```python
from build123d import *

# Parameters (mm, degrees)
SKETCH2_W                = 20
SKETCH2_H                = 5
BOSS_EXTRUDE1_DEPTH      = 10
SKETCH4_R                = 2
BOSS_EXTRUDE2_DEPTH      = 3.333333333
BOSS_EXTRUDE3_START      = -3.333333333
SKETCH5_R                = 2
BOSS_EXTRUDE3_DEPTH      = 3.333333333
BOSS_EXTRUDE4_DEPTH      = 1.5
BOSS_EXTRUDE4_DEPTH_BACK = 1.5
SKETCH7_R                = 2
BOSS_EXTRUDE5_DEPTH      = 1.5
BOSS_EXTRUDE5_DEPTH_BACK = 1.5
CUT_EXTRUDE1_DEPTH       = 27.57654043


with BuildPart() as part:
    # Sketch2 → Boss-Extrude1 (new body)
    with BuildSketch(Plane(origin=(0, 0, 0), x_dir=(0, 0, -1), z_dir=(1, 0, 0))):
        with Locations((10, 2.5)):
            Rectangle(SKETCH2_W, SKETCH2_H)
    extrude(amount=BOSS_EXTRUDE1_DEPTH)

    # Sketch4 → Boss-Extrude2 (add)
    with BuildSketch(Plane(origin=(10, 0, 0), x_dir=(0, 0, -1), z_dir=(1, 0, 0))):
        with BuildLine():
            Line((-2.5, 5), (0, 5))
            Line((0, 5), (0, 2.5))
            ThreePointArc((0, 2.5), (-4.267766953, 0.732233047), (-2.5, 5))
        make_face()
        with Locations((-2.5, 2.5)):
            Circle(SKETCH4_R, mode=Mode.SUBTRACT)
    extrude(amount=-BOSS_EXTRUDE2_DEPTH)

    # Sketch5 → Boss-Extrude3 (add)
    with BuildSketch(Plane.ZY.offset(BOSS_EXTRUDE3_START)):
        with BuildLine():
            Line((2.5, 5), (0, 5))
            Line((0, 5), (0, 2.5))
            ThreePointArc((0, 2.5), (4.267766953, 0.732233047), (2.5, 5))
        make_face()
        with Locations(Location((2.5, 2.5, 0), (0, 0, 180))):
            Circle(SKETCH5_R, mode=Mode.SUBTRACT)
    extrude(amount=BOSS_EXTRUDE3_DEPTH)

    # Sketch7 → Boss-Extrude4 (add, two sides: drawn at the far end of the back side and taken through both)
    with BuildSketch(Plane(origin=(5, 0, 0), x_dir=(0, 0, -1), z_dir=(1, 0, 0)).offset(-BOSS_EXTRUDE4_DEPTH_BACK)):
        with BuildLine():
            Line((20, 5), (22.5, 5))
            ThreePointArc((22.5, 5), (24.267766953, 0.732233047), (20, 2.5))
            Line((20, 2.5), (20, 5))
        make_face()
        with Locations((22.5, 2.5)):
            Circle(SKETCH7_R, mode=Mode.SUBTRACT)
    extrude(amount=BOSS_EXTRUDE4_DEPTH + BOSS_EXTRUDE4_DEPTH_BACK)

    # Sketch8 → Boss-Extrude5 (add, two sides: drawn at the far end of the back side and taken through both)
    with BuildSketch(Plane(origin=(5, 0, 0), x_dir=(0, 0, -1), z_dir=(1, 0, 0)).offset(-BOSS_EXTRUDE5_DEPTH_BACK)):
        with BuildLine():
            Line((0, 5), (2, 5))
            Line((2, 5), (5.2, 5))
            Line((5.2, 5), (5.2, 5.04))
            add(Edge.make_bspline(
                [(2, 6.25), (2.633677282, 6.25), (3.485069852, 5.13334343), (4.685132782, 5.04), (5.2, 5.04)],
                knots=[0, 0, 0, 0, 0.555540961, 1, 1, 1, 1], degree=3))
            Line((2, 6.25), (-8, 6.25))
            Line((-8, 6.25), (-8, 5))
            Line((-8, 5), (0, 5))
        make_face()
    extrude(amount=BOSS_EXTRUDE5_DEPTH + BOSS_EXTRUDE5_DEPTH_BACK)

    # Sketch9 → Cut-Extrude1 (cut, through all)
    with BuildSketch(Plane.ZY.offset(-3.5)):
        Polygon((8, 6.25), (5.838024107, 6.25), (5.838024107, 5.183121739), (2.5, 5.183121739), (2.5, 5), (8, 5), align=None)
    extrude(amount=-CUT_EXTRUDE1_DEPTH, mode=Mode.SUBTRACT)


solid = part.part
```
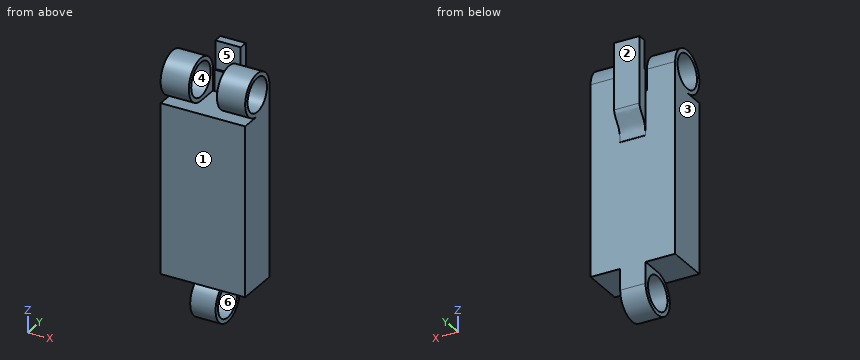
The model under review builds one solid part; all positions refer to its coordinate system, in mm. Face numbers are marked on the shaded views. A direction names the side the tool comes from. Give positions to 0.01 mm unless a question says otherwise; leave off trailing zeros. Write each loop counter-clockwise with the first axis right and the second up, starting at its lowest first coordinate (ties: lowest second). Pieces come first, ordered by that corner, then holes. Notation, with made-up numbers: (57.5, 72.5) -> (76.5, 72.5) arc R14 ccw to (76.5, 80.5) -> close; hole circle Ø6 at (85, -14). An arc over 180 degrees is marked (long way). Answer in a Markdown table with one row per item.
1) Add section A-A on y = 4. State the section outline as (x, z) points.
Worked answers:
| item | result |
|---|---|
| outline | (0, -20) -> (3.5, -20) -> (3.5, -21.18) -> (6.5, -21.18) -> (6.5, -20) -> (10, -20) -> (10, 1.18) -> (6.67, 1.18) -> (6.67, 0) -> (3.33, 0) -> (3.33, 1.18) -> (0, 1.18) -> close; (0, 3.82) -> (3.33, 3.82) -> (3.33, 4.5) -> (0, 4.5) -> close; (3.5, -24.5) -> (6.5, -24.5) -> (6.5, -23.82) -> (3.5, -23.82) -> close; (6.67, 3.82) -> (10, 3.82) -> (10, 4.5) -> (6.67, 4.5) -> close |
2) Clearance check with flat-ended pins moving along their axes: P1, Ø1.5, axis at x = 3, y = 1.5, coming from the +Z side; P2, Ø3.5, axis at x = 4.5, z = 4.5, coming from the -Y side; P3, Ø5, axis at x = 2.5, z = -12.5, coming from the +Y side. State where each tip first meets the part, or that it passes through.
Worked answers:
| item | result |
|---|---|
| P1 | z = 4.99 |
| P2 | y = 0.1 |
| P3 | y = 5 |
3) Mouldability with a two-part tool opening along Y and no side actions: class the marked faces 1, 2, 3 and 4 as +Y half, -Y half, draft (parallel to the pull), parting line (faces both ways), or undercut.
Worked answers:
| item | result |
|---|---|
| face 1 | -Y half |
| face 2 | +Y half |
| face 3 | draft |
| face 4 | undercut |
4) Add section D-D on z = -7. State the section outline as (x, y) points, plus the area to 3 significant figures.
Worked answers:
| item | result |
|---|---|
| outline | (0, 0) -> (10, 0) -> (10, 5) -> (0, 5) -> close |
| area | 50.0 mm² |
5) For L1, parallel to Y at x = 1.45, z = 2.5; L2, parallel to Y at x = 8, z = -3; L3, parallel to Y at x = 5.75, z = 3.5, list the stretches that pass through material, from the lowest coordinate up. Write a range as [from, to].
Worked answers:
| item | result |
|---|---|
| L1 | [0, 0.5], [4.5, 5] |
| L2 | [0, 5] |
| L3 | [5.18, 6.25] |
6) Add section C-C on y = 1. State the section outline as (x, z) points, plus the area to 3 significant figures.
Worked answers:
| item | result |
|---|---|
| outline | (0, -20) -> (10, -20) -> (10, 0) -> (0, 0) -> close; (0, 0.5) -> (3.33, 0.5) -> (3.33, 1.18) -> (0, 1.18) -> close; (0, 3.82) -> (3.33, 3.82) -> (3.33, 4.5) -> (0, 4.5) -> close; (3.5, -24.5) -> (6.5, -24.5) -> (6.5, -23.82) -> (3.5, -23.82) -> close; (3.5, -21.18) -> (6.5, -21.18) -> (6.5, -20.5) -> (3.5, -20.5) -> close; (6.67, 0.5) -> (10, 0.5) -> (10, 1.18) -> (6.67, 1.18) -> close; (6.67, 3.82) -> (10, 3.82) -> (10, 4.5) -> (6.67, 4.5) -> close |
| area | 213 mm² |
7) Tool access review of the marked faces 5 and 6: name each direction out of +Z, -Z, +X, -X, +Y, -Y from which nothing blocks a thin tool from reaching the whole face with its end or side.
Worked answers:
| item | result |
|---|---|
| face 5 | +Z, +X, -X, -Y |
| face 6 | +X, -X |
8) Add section B-B on z = -22. State the section outline as (x, y) points.
Worked answers:
| item | result |
|---|---|
| outline | (3.5, 0.05) -> (6.5, 0.05) -> (6.5, 0.56) -> (3.5, 0.56) -> close; (3.5, 4.44) -> (6.5, 4.44) -> (6.5, 5) -> (3.5, 5) -> close |
